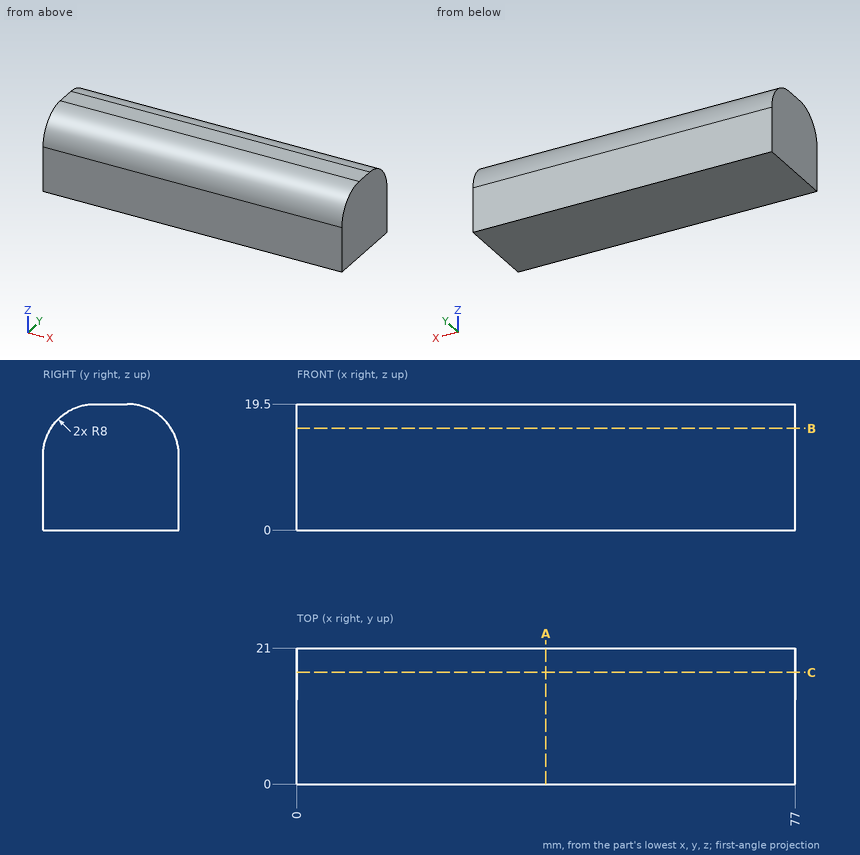
Could you check a few things on this drawing? It's one solid part, dimensions in mm from its lowest x, y, z. Round coordinates to 2 decimals unless told otherwise and drop trailing zeros. Order: outer loops, then holes, each group sorted by start corner. A loop starts at its lowest first (then second) coordinate and runs counter-clockwise, first axis right, second up. Notation, with made-up numbers: M 76.25,-34.75 L 82.25,-34.75 A32 cw 82.25,-1.75 Z; hole C 71.25,-30 d1. An arc over 180 degrees is marked long. Return JSON: item names as keys, results as strings. Group by question number.
1. Please list where these lines run through material, in increasing order: probe 1 along Z at (x, y) = (10.5, 13.25); probe 2 along Y at (x, z) = (23.5, 12.75); probe 3 along Y at (x, z) = (69, 13.25).
2. If we section it at C-C on y = 17.25: List the corners of the cut face in (x, z) for me, then the cut area to 3 significant figures.
3. If we section it at A-A on x = 38.5: List the corners of the cut face in (y, z) for me.
4. I'm going to push flat-ended pins straight in: pin 1 Ø6 at (x, y) = (55.5, 14.5) entering from +Z; pin 2 Ø5 at (x, z) = (42, 16.5) entering from -Y; pin 3 Ø6 at (x, y) = (67.5, 3.5) entering from +Z. Where does each tip first touch, or does it pass through?
5. If we section it at B-B on z = 15.75: List the corners of the cut face in (x, y) for me.
Reply:
{
 "1": {"probe 1": "0 to 19.5", "probe 2": "0.1 to 20.9", "probe 3": "0.19 to 20.81"},
 "2": {"outline": "M 0,0 L 77,0 L 77,18.28 L 0,18.28 Z", "area": "1,410 mm^2"},
 "3": {"outline": "M 0,0 L 21,0 L 21,11.5 A8 ccw 13,19.5 L 8,19.5 A8 ccw 0,11.5 Z"},
 "4": {"pin 1": "z = 19.5", "pin 2": "y = 0.4", "pin 3": "z = 19.36"},
 "5": {"outline": "M 0,1.22 L 77,1.22 L 77,19.78 L 0,19.78 Z"}
}
